Geometry check sheet. Reference: the model listing, model coordinates, mm. A direction names the side the tool comes from. Give positions to 0.01 mm unless a question says otherwise; leave off trailing zeros. Order: outer loops, then holes, each group sorted by start corner. A loop starts at its lowest first (then second) coordinate and runs counter-clockwise, first axis right, second up. Notation, with made-up numbers: (65, 28.5) - (111, 28.5) arc R18 ccw to (111, 38.5) - close; hole circle Ø8 at (45.5, 4). An arc over 180 degrees is marked (long way). Put each result on its own line as item: value. Start each with the question number.
```python
from build123d import *

# Parameters (mm, degrees)
F0_R     = 11
F1_DEPTH = 9


with BuildPart() as f1:
    # F0 (on Top) → F1 (new body)
    with BuildSketch(Plane.XY):
        with BuildLine():
            ThreePointArc((-36.851079, 9.464021), (-39.389584, -4.277113), (-36.232757, -17.889505))
            ThreePointArc((-36.232757, -17.889505), (-35.619676, -19.115828), (-34.958043, -20.316652))
            ThreePointArc((-34.958043, -20.316652), (-22.102923, -28.572601), (-8.67895, -21.277965))
            ThreePointArc((-8.67895, -21.277965), (1.696424, -16.308632), (11.338573, -22.583312))
            ThreePointArc((11.338573, -22.583312), (12.196181, -30.664961), (7.987033, -37.617055))
            ThreePointArc((7.987033, -37.617055), (23.55354, -32.423652), (34.921925, -20.58949))
            ThreePointArc((34.921925, -20.58949), (35.19653, -6.086622), (23.066393, 1.867519))
            ThreePointArc((23.066393, 1.867519), (13.575138, 8.36819), (14.188096, 19.855876))
            ThreePointArc((14.188096, 19.855876), (20.235163, 25.094459), (28.21375, 25.687702))
            ThreePointArc((28.21375, 25.687702), (15.932878, 36.571991), (0, 40.50022))
            ThreePointArc((0, 40.50022), (-12.697154, 33.486601), (-13.520574, 19.004523))
            ThreePointArc((-13.520574, 19.004523), (-13.750641, 6.869394), (-24.594523, 1.417373))
            ThreePointArc((-24.594523, 1.417373), (-31.129245, 3.546576), (-35.603177, 8.763859))
            ThreePointArc((-35.603177, 8.763859), (-36.022944, 9.741554), (-36.359555, 10.750902))
            Line((-36.359555, 10.750902), (-36.851079, 9.464021))
        make_face()
        with Locations((-21.232757, -13.068097)):
            Circle(F0_R, mode=Mode.SUBTRACT)
        Circle(F0_R, mode=Mode.SUBTRACT)
        with Locations((22.986825, -13.132481)):
            Circle(F0_R, mode=Mode.SUBTRACT)
        with Locations((0, 25.50022)):
            Circle(F0_R, mode=Mode.SUBTRACT)
    extrude(amount=F1_DEPTH)


solid = f1.part
```
Item 1: Gauge pin test, flat ends, axial feed: pin 1 Ø2 at (x, z) = (-7.5, 1.5) entering from +Y; pin 2 Ø3 at (y, z) = (14.5, 4) entering from +X; pin 3 Ø2 at (x, z) = (10, 5.5) entering from +Y. Record the tip position at first contact, or that the pin passes through.
Item 2: Cross-section at B-B (x = -2). Enter the section's corners in (y, z), and give its area (3 significant figures).
Item 3: Thickness scan on line 1 along Y through (x, z) = (0, 2.25); line 2 along Y through (x, z) = (-6.5, 2.25); line 3 along Y through (x, z) = (10, 8). Record the ranges inside material, lowest first.
Item 4: Cross-section at A-A (y = 31). Enter the section's corners in (x, z), and give its area (3 significant figures).
Item 5: Set-up check for faces 1 (the face through (-13.657, 7.021, 4.437)), 2 (the face through (-36.02, 9.73, 4.44)), 3 (the face through (-1, -13, 9)): record each of +Z, -Z, +X, -X, +Y, -Y from which the full face is reachable in a straight line by a thin tool's end or side.
Item 6: Release check for a two-part mould opening along X. For faces 4 (the face through (1.53, -16.3, 4.44)), 5 (the face through (23.357, -32.547, 4.437)), 6 (the face through (-39.393, -4.08, 4.437)), 7 (the face through (-1, -13, 0)) record: +X half, -X half, draft (parallel to the pull), parting line (faces both ways), or undercut.
Item 7: Cross-section at D-D (z = 7). Enter the section's corners in (x, y).
Item 8: Cross-section at C-C (x = 30). Enter the section's corners in (y, z).
Recorded:
1. pin 1: stops at y = 39.02
1. pin 2: stops at x = 12.62
1. pin 3: stops at y = 39.3
2. outline: (-16.66, 0) - (-10.82, 0) - (-10.82, 9) - (-16.66, 9) - close; (10.82, 0) - (14.68, 0) - (14.68, 9) - (10.82, 9) - close; (36.32, 0) - (40.37, 0) - (40.37, 9) - (36.32, 9) - close
2. area: 124 mm^2
3. line 1: y = -16.32 to -11, 11 to 14.5, 36.5 to 40.5
3. line 2: y = -18.93 to -8.87, 8.87 to 16.63, 34.37 to 39.02
3. line 3: y = -37.4 to -35.47, -20.56 to -4.58, 4.58 to 20.92, 30.08 to 39.01
4. outline: (-13.96, 0) - (-9.53, 0) - (-9.53, 9) - (-13.96, 9) - close; (9.53, 0) - (23.69, 0) - (23.69, 9) - (9.53, 9) - close
4. area: 167 mm^2
5. face 1: +Z, -Z
5. face 2: +Z, -Z, +Y
5. face 3: +Z, +X, -X, +Y, -Y
6. face 4: undercut
6. face 5: +X half
6. face 6: -X half
6. face 7: draft
7. outline: (-36.85, 9.46) arc R34.28 ccw to (-36.23, -17.89) arc R34.28 ccw to (-34.96, -20.32) arc R15 ccw to (-8.68, -21.28) arc R11.75 cw to (11.34, -22.58) arc R12.72 cw to (7.99, -37.62) arc R34.28 ccw to (34.92, -20.59) arc R15 ccw to (23.07, 1.87) arc R11.75 cw to (14.19, 19.86) arc R12.72 cw to (28.21, 25.69) arc R34.28 ccw to (0, 40.5) arc R15 ccw to (-13.52, 19) arc R11.75 cw to (-24.59, 1.42) arc R12.72 cw to (-35.6, 8.76) arc R12.72 cw to (-36.36, 10.75) - close; hole circle Ø22 at (-21.23, -13.07); hole circle Ø22 at (0, 0); hole circle Ø22 at (0, 25.5); hole circle Ø22 at (22.99, -13.13)
8. outline: (-27.15, 0) - (-21.61, 0) - (-21.61, 9) - (-27.15, 9) - close; (-4.66, 0) - (-0.44, 0) - (-0.44, 9) - (-4.66, 9) - close
